Autodesk Inventor part; units mm, degrees
ref_plane "YZ Plane" through (0, 0, 0) normal (1, 0, 0) x (0, 1, 0)
ref_plane "XZ Plane" through (0, 0, 0) normal (0, 1, 0) x (-1, 0, 0)
ref_plane "XY Plane" through (0, 0, 0) normal (0, 0, 1) x (1, 0, 0)
sketch "스케치1" plane through (0, 0, 0) normal (0, 1, 0) x (-1, 0, 0)
  line L0 (-24.9446, -24.9446) -> (24.9446, -24.9446)
  line L1 (24.9446, -24.9446) -> (24.9446, 24.9446)
  line L2 (24.9446, 24.9446) -> (-24.9446, 24.9446)
  line L3 (-24.9446, 24.9446) -> (-24.9446, -24.9446)
  line L4 (-24.9446, -24.9446) -> (24.9446, 24.9446) construction
  line L5 (24.9446, -24.9446) -> (-24.9446, 24.9446) construction
  line L6 (-28.1446, -28.1446) -> (28.1446, -28.1446)
  line L7 (28.1446, -28.1446) -> (28.1446, 28.1446)
  line L8 (28.1446, 28.1446) -> (-28.1446, 28.1446)
  line L9 (-28.1446, 28.1446) -> (-28.1446, -28.1446)
  line L10 (-28.1446, -28.1446) -> (28.1446, 28.1446) construction
  line L11 (28.1446, -28.1446) -> (-28.1446, 28.1446) construction
  point P0 (0, 0)
  dimension "d0" = 70.554
  dimension "d1" = 3.2
extrude "돌출1" add sketch "스케치1" along normal blind 3.7 contours L3 L2 L1 L0 | L9 L8 L7 L6
sketch "스케치2" plane through (0, 3.7, 0) normal (0, 1, 0) x (1, 0, 0)
  line L0 (-28.1446, 28.1446) -> (-28.1446, -28.1446)
  line L1 (-28.1446, -28.1446) -> (28.1446, -28.1446)
  line L2 (28.1446, -28.1446) -> (28.1446, 28.1446)
  line L3 (28.1446, 28.1446) -> (-28.1446, 28.1446)
  line L4 (26.5446, 26.5446) -> (-26.5446, 26.5446)
  line L5 (-26.5446, 26.5446) -> (-26.5446, -26.5446)
  line L6 (-26.5446, -26.5446) -> (26.5446, -26.5446)
  line L7 (26.5446, -26.5446) -> (26.5446, 26.5446)
  line L8 (26.5446, 26.5446) -> (-26.5446, -26.5446) construction
  line L9 (-26.5446, 26.5446) -> (26.5446, -26.5446) construction
  line L10 (24.5446, 24.5446) -> (-24.5446, 24.5446)
  line L11 (-24.5446, 24.5446) -> (-24.5446, -24.5446)
  line L12 (-24.5446, -24.5446) -> (24.5446, -24.5446)
  line L13 (24.5446, -24.5446) -> (24.5446, 24.5446)
  line L14 (24.5446, 24.5446) -> (-24.5446, -24.5446) construction
  line L15 (-24.5446, 24.5446) -> (24.5446, -24.5446) construction
  point P0 (0, 0)
  point P1 (0, 28.1446)
  point P2 (-28.1446, 0)
  dimension "d4" = 1.6
  dimension "d5" = 2
extrude "돌출2" cut sketch "스케치2" against normal blind 1.2 contours L7 L6 L5 L4 | L13 L12 L11 L10
sketch "스케치3" plane through (0, 2.5, 0) normal (0, 1, 0) x (1, 0, 0)
  line L0 (24.5446, 24.5446) -> (-24.5446, 24.5446)
  line L1 (-24.5446, 24.5446) -> (-24.5446, -24.5446)
  line L2 (-24.5446, -24.5446) -> (24.5446, -24.5446)
  line L3 (24.5446, -24.5446) -> (24.5446, 24.5446)
  line L4 (24.5446, 24.5446) -> (-24.5446, -24.5446) construction
  line L5 (-24.5446, 24.5446) -> (24.5446, -24.5446) construction
  line L6 (-26.5446, -26.5446) -> (-26.5446, 26.5446)
  point P0 (0, 0)
  dimension "d8" = 2
extrude "돌출3" add sketch "스케치3" along normal blind 0.6
fillet "모깎기1" radius 1.2 8 edges at (0, 3.7, 28.1446) (28.1446, 3.7, 0) (0, 3.7, -28.1446) (-28.1446, 3.7, 0) (-28.1446, 0, 0) (0, 0, 28.1446) (28.1446, 0, 0) (0, 0, -28.1446)
sketch "스케치11" plane through (0, 0, 0) normal (0, -1, 0) x (1, 0, 0)
  circle A0 centre (0, 0) radius 12.7
  dimension "d50" = 25.4
extrude "돌출11" add sketch "스케치11" along normal blind 10.16
sketch "스케치12" plane through (0, -10.16, 0) normal (0, -1, 0) x (1, 0, 0)
  circle A0 centre (0, 0) radius 4.5
  line L0 (-2.5981, 4.5) -> (2.5981, 4.5)
  line L1 (2.5981, 4.5) -> (5.1962, 0)
  line L2 (5.1962, 0) -> (2.5981, -4.5)
  line L3 (2.5981, -4.5) -> (-2.5981, -4.5)
  line L4 (-2.5981, -4.5) -> (-5.1962, 0)
  line L5 (-5.1962, 0) -> (-2.5981, 4.5)
  point P0 (-3.8971, 2.25)
  point P1 (-3.8971, -2.25)
  point P2 (0, 4.5)
  point P3 (0, -4.5)
  point P4 (3.8971, -2.25)
  point P5 (3.8971, 2.25)
  dimension "d53" = 9
extrude "돌출12" cut sketch "스케치12" against normal blind 12
sketch "스케치13" plane through (0, 0, 0) normal (0, -1, 0) x (1, 0, 0)
  circle A0 centre (-18, 0) radius 5
  circle A1 centre (-9, -15.5885) radius 5
  circle A2 centre (9, -15.5885) radius 5
  circle A3 centre (18, 0) radius 5
  circle A4 centre (9, 15.5885) radius 5
  circle A5 centre (-9, 15.5885) radius 5
  point P0 (0, 0)
  dimension "d58" = 10
  dimension "d59" = 18
  dimension "d62" = 360
extrude "돌출13" cut sketch "스케치13" against normal up to surface (3.1 mm away)
sketch "스케치16" plane through (0, 1.84, 0) normal (0, -1, 0) x (1, 0, 0)
  line L0 (-2.0207, 3.5) -> (2.0207, 3.5)
  line L1 (2.0207, 3.5) -> (4.0415, 0)
  line L2 (4.0415, 0) -> (2.0207, -3.5)
  line L3 (2.0207, -3.5) -> (-2.0207, -3.5)
  line L4 (-2.0207, -3.5) -> (-4.0415, 0)
  line L5 (-4.0415, 0) -> (-2.0207, 3.5)
  line L6 (-5.1962, 0) -> (-2.5981, 4.5)
  line L7 (-2.5981, 4.5) -> (2.5981, 4.5)
  line L8 (-5.1962, 0) -> (-2.5981, 4.5)
  line L9 (-2.5981, -4.5) -> (-5.1962, 0)
  line L10 (2.5981, -4.5) -> (-2.5981, -4.5)
  line L11 (5.1962, 0) -> (2.5981, -4.5)
  line L12 (2.5981, 4.5) -> (5.1962, 0)
  point P0 (0, 0)
  point P1 (0, 0)
  dimension "d84" = 1
extrude "돌출14" add sketch "스케치16" along normal blind 8.5
fillet "모깎기2" radius 0.5 6 edges at (-3.8971, -10.16, 2.25) (0, -10.16, 4.5) (3.8971, -10.16, 2.25) (3.8971, -10.16, -2.25) (0, -10.16, -4.5) (-3.8971, -10.16, -2.25)
equation "\"d73\" = 55deg"
properties part number "OV-PAM_n_4_bottom"
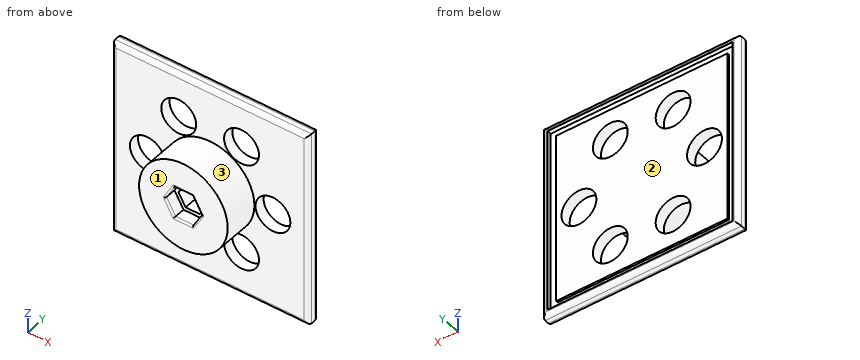
Build history of the part. All positions in model axes, mm. Face numbers are marked on the shaded views. Coordinates: 2 decimals unless noted, no trailing zeros. Write each loop counter-clockwise with the first axis right and the second up, starting at its lowest first coordinate (ties: lowest second). Pieces come first, ordered by that corner, then holes.
1. Band-saw the part on B-B, the plane y = -3. Give the cut face in (x, z), and give its area (3 significant figures).
Answer block:
outline: circle Ø25.4 at (0, 0); hole (-4.04, 0) - (-2.02, -3.5) - (2.02, -3.5) - (4.04, 0) - (2.02, 3.5) - (-2.02, 3.5) - close
area: 464 mm2
2. Drill centre lines: probe 1 along Z at (x, y) = (9, 1.7); probe 2 along Z at (x, y) = (18, 2); probe 3 along Y at (x, z) = (14.5, -17). Where is each one in solid material? Low to high.
Answer block:
probe 1: z = -28.14 to -20.59, -10.59 to 10.59, 20.59 to 28.14
probe 2: z = -28.14 to -5, 5 to 28.14
probe 3: y = 0 to 3.1
3. Band-saw the part on C-C, the plane z = -19.5. Give the cut face in (x, y).
Answer block:
outline: (-28.14, 1.2) arc R1.2 ccw to (-26.94, 0) - (-12.11, 0) - (-12.11, 3.1) - (-24.54, 3.1) - (-24.54, 2.5) - (-26.54, 2.5) - (-26.54, 3.7) - (-26.94, 3.7) arc R1.2 ccw to (-28.14, 2.5) - close; (-5.89, 0) - (5.89, 0) - (5.89, 3.1) - (-5.89, 3.1) - close; (12.11, 0) - (26.94, 0) arc R1.2 ccw to (28.14, 1.2) - (28.14, 2.5) arc R1.2 ccw to (26.94, 3.7) - (26.54, 3.7) - (26.54, 2.5) - (24.54, 2.5) - (24.54, 3.1) - (12.11, 3.1) - close
4. Band-saw the part on A-A, the plane x = -15. Give the cut face in (y, z).
Answer block:
outline: (0, -26.94) arc R1.2 ccw to (1.2, -28.14) - (2.5, -28.14) arc R1.2 ccw to (3.7, -26.94) - (3.7, -26.54) - (2.5, -26.54) - (2.5, -24.54) - (3.1, -24.54) - (3.1, -4) - (0, -4) - close; (0, 4) - (3.1, 4) - (3.1, 24.54) - (2.5, 24.54) - (2.5, 26.54) - (3.7, 26.54) - (3.7, 26.94) arc R1.2 ccw to (2.5, 28.14) - (1.2, 28.14) arc R1.2 ccw to (0, 26.94) - close
5. Band-saw the part on D-D, the plane x = 18. Give the cut face in (y, z).
Answer block:
outline: (0, -26.94) arc R1.2 ccw to (1.2, -28.14) - (2.5, -28.14) arc R1.2 ccw to (3.7, -26.94) - (3.7, -26.54) - (2.5, -26.54) - (2.5, -24.54) - (3.1, -24.54) - (3.1, -5) - (0, -5) - close; (0, 5) - (3.1, 5) - (3.1, 24.54) - (2.5, 24.54) - (2.5, 26.54) - (3.7, 26.54) - (3.7, 26.94) arc R1.2 ccw to (2.5, 28.14) - (1.2, 28.14) arc R1.2 ccw to (0, 26.94) - close
6. Pull direction X, two halves, no side cores. Call the marked faces 1, 2 and 3: released by +X, released by -X, zero draft, split by the parting line, or undercut.
Answer block:
face 1: zero draft
face 2: undercut
face 3: split by the parting line
7. Drop flat-ended pins along their axis: pin 1 (3 mm diameter, centred on x = -20.5, z = 4, fed in from +Y); pin 2 (1 mm diameter, centred on y = 3.5, z = -8, fed in from -X); pin 3 (0.5 mm diameter, centred on y = 3, z = 10.5, fed in from +X). Give the stop position or say it passes through.
Answer block:
pin 1: stops at y = 3.1
pin 2: stops at x = -28.04
pin 3: stops at x = 28.12
